Check sheet for the modelled part. Datum: model origin and axes. Units: mm. A direction names the side the tool comes from. Give positions to 0.01 mm unless a question says otherwise; leave off trailing zeros. Write each loop counter-clockwise with the first axis right and the second up, starting at its lowest first coordinate (ties: lowest second). Pieces come first, ordered by that corner, then holes. Notation, with made-up numbers: (-37, -1) -> (-32, -1) arc R10 cw to (-32, 12) -> close; hole circle Ø6 at (65.5, -24). An arc over 180 degrees is marked (long way). Answer as a JSON object with one key per item and string values.
Autodesk Inventor part; units mm, degrees
ref_plane "hhpsjc_r_XY" through (0, 0, 0) normal (0, 1, 0) x (1, 0, 0)
ref_plane "hhpsjc_r_YZ" through (0, 0, 0) normal (1, 0, 0) x (0, 0, -1)
ref_plane "hhpsjc_r_ZX" through (0, 0, 0) normal (0, 0, -1) x (0, 1, 0)
sketch "Sketch_1" plane through (0, 0, 0) normal (0, 0, 1) x (1, 0, 0)
  line L0 (0, -16) -> (0, 16)
  line L1 (0, 16) -> (5, 16)
  line L2 (5, 16) -> (5, -16)
  line L3 (5, -16) -> (0, -16)
  line L4 (0, -16) -> (0, 16)
revolve "Revolution1" add sketch "Sketch_1" angle 360 about axis through (0, -16, 0) along (0, -1, 0)
sketch "Sketch_2" plane through (0, 0, 0) normal (0, 1, 0) x (-1, 0, 0)
  line L0 (0, 1) -> (-16, 1)
  arc A0 (-16, 1) -> (-18, -5) centre (-8, -5) ccw
  line L1 (-18, -5) -> (0, -5)
  line L2 (0, -5) -> (0, 1)
extrude "Extrusion1" add sketch "Sketch_2" along normal mid plane 32
sketch "Sketch_4" plane through (18, 0, 0) normal (1, 0, 0) x (0, 0, -1)
  line L0 (-5, -32) -> (10, -32)
  line L1 (10, -32) -> (10, 32)
  line L2 (10, 32) -> (-5, 32)
  line L3 (-5, 32) -> (-5, -32)
  line L4 (-1, 14) -> (-1, -14)
  arc A0 (-1, -14) -> (5, -16) centre (5, -6) ccw
  line L5 (5, -16) -> (5, 16)
  arc A1 (5, 16) -> (-1, 14) centre (5, 6) ccw
extrude "Extrusion2" cut sketch "Sketch_4" against normal blind 13
sketch "Sketch_6" plane through (0, 0, -5) normal (0, 0, 1) x (1, 0, 0)
  circle A0 centre (10.5, 12) radius 2.75
extrude "Extrusion3" add sketch "Sketch_6" against normal blind 4
sketch "Sketch_5" plane through (0, 0, -5) normal (0, 0, 1) x (1, 0, 0)
  circle A0 centre (10.5, -12) radius 2.75
extrude "Extrusion4" add sketch "Sketch_5" against normal blind 4
sketch "Sketch_7" plane through (10.5, 0, 0) normal (1, 0, 0) x (0, 0, -1)
  line L0 (5, 0) -> (-1, 0)
  line L1 (-1, 0) -> (-1, 5.5)
  line L2 (-1, 5.5) -> (1.75, 2.75)
  line L3 (1.75, 2.75) -> (5, 2.75)
  line L4 (5, 2.75) -> (5, 0)
  line L5 (5, 0) -> (-1, 0)
revolve "Revolution2" cut sketch "Sketch_7" angle 360 about axis through (10.5, 0, -5) along (0, 0, -1)
sketch "Sketch_8" plane through (0, 0, 0) normal (0, 0, 1) x (1, 0, 0)
  line L0 (0, -16) -> (0, 16)
  line L1 (0, 16) -> (2.5, 16)
  line L2 (2.5, 16) -> (2.5, -16)
  line L3 (2.5, -16) -> (0, -16)
  line L4 (0, -16) -> (0, 16)
revolve "Revolution3" cut sketch "Sketch_8" angle 360 about axis through (0, -16, 0) along (0, -1, 0)
sketch "Sketch_3" plane through (0, 0, 0) normal (0, 0, 1) x (1, 0, 0)
  line L0 (-36, -36) -> (36, -36)
  line L1 (36, -36) -> (36, 36)
  line L2 (36, 36) -> (-36, 36)
  line L3 (-36, 36) -> (-36, -36)
  line L4 (-5, -16) -> (14, -16)
  arc A0 (14, -16) -> (18, -12) centre (14, -12) ccw
  line L5 (18, -12) -> (18, 12)
  arc A1 (18, 12) -> (14, 16) centre (14, 12) ccw
  line L6 (14, 16) -> (-5, 16)
  line L7 (-5, 16) -> (-5, 5.5333)
  line L8 (-5, 5.5333) -> (5, 5.5333)
  line L9 (5, 5.5333) -> (5, -5.5333)
  line L10 (5, -5.5333) -> (-5, -5.5333)
  line L11 (-5, -5.5333) -> (-5, -16)
extrude "Extrusion5" cut sketch "Sketch_3" along normal mid plane 10
ref_plane "hhpsjc_r_XY" through (0, 0, 0) normal (0, 1, 0) x (1, 0, 0)
ref_plane "hhpsjc_r_YZ" through (0, 0, 0) normal (1, 0, 0) x (0, 0, -1)
ref_plane "hhpsjc_r_ZX" through (0, 0, 0) normal (0, 0, -1) x (0, 1, 0)
ref_plane "hole2_to_bolt_XY" through (10.5, 0, 1) normal (0, 0, 1) x (1, 0, 0)
ref_plane "hole2_to_bolt_YZ" through (10.5, 0, 1) normal (1, 0, 0) x (0, 1, 0)
ref_plane "hole2_to_bolt_ZX" through (10.5, 0, 1) normal (0, 1, 0) x (0, 0, 1)
ref_plane "nut2_to_bolt_XY" through (10.5, 0, -7) normal (0, 0, 1) x (1, 0, 0)
ref_plane "nut2_to_bolt_YZ" through (10.5, 0, -7) normal (1, 0, 0) x (0, 1, 0)
ref_plane "nut2_to_bolt_ZX" through (10.5, 0, -7) normal (0, 1, 0) x (0, 0, 1)
properties part number "HHPSJC5-r"
1. Mould release check, pull along Y, two halves, no side actions. Record for faces 6 (the face through (2, 16, -2)), 7 (the face through (2, -16, -2)), 8 (the face through (-0.54, -10.84, -2.44)), 9 (the face through (13.35, -0.63, -1.58)): released by +Y, released by -Y, zero draft, split by the parting line, or undercut.
Determined:
{"face 6": "released by +Y", "face 7": "released by -Y", "face 8": "zero draft", "face 9": "undercut"}
2. Sectioned sample at B-B, the plane z = -1. Enter the section's corners in (x, y).
Determined:
{"outline": "(-4.9, -16) -> (-2.29, -16) -> (-2.29, -5.53) -> (-4.9, -5.53) -> close; (-4.9, 5.53) -> (-2.29, 5.53) -> (-2.29, 16) -> (-4.9, 16) -> close; (2.29, -16) -> (5, -16) -> (5, -15.17) -> (16.45, -15.17) arc R4 ccw to (17.17, -14.45) -> (17.17, 14.45) arc R4 ccw to (16.45, 15.17) -> (5, 15.17) -> (5, 16) -> (2.29, 16) -> (2.29, 5.53) -> (5, 5.53) -> (5, -5.53) -> (2.29, -5.53) -> close; hole circle Ø7 at (10.5, 0)"}
3. Sectioned sample at A-A, the plane x = 4. Enter the section's corners in (y, z), plus the area to 3 significant figures.
Determined:
{"outline": "(-16, -5) -> (-5.53, -5) -> (-5.53, 3) -> (-16, 3) -> close; (5.53, -5) -> (16, -5) -> (16, 3) -> (5.53, 3) -> close", "area": "167 mm^2"}
4. Sectioned sample at D-D, the plane x = -1.75. Enter the section's corners in (y, z).
Determined:
{"outline": "(-16, -4.68) -> (-5.53, -4.68) -> (-5.53, -1.79) -> (-16, -1.79) -> close; (-16, 1.79) -> (-5.53, 1.79) -> (-5.53, 4.68) -> (-16, 4.68) -> close; (5.53, -4.68) -> (16, -4.68) -> (16, -1.79) -> (5.53, -1.79) -> close; (5.53, 1.79) -> (16, 1.79) -> (16, 4.68) -> (5.53, 4.68) -> close"}
5. Scan lines: L1, parallel to Z at x = 0, y = 8; L2, parallel to Y at x = -2.5, z = -2.5; L3, parallel to X at y = 0, z = -3.05. Record each from-to range of solid material in increasing order. Write a range as [from, to].
Determined:
{"L1": "[-5, -2.5], [2.5, 5]", "L2": "[-16, -5.53], [5.53, 16]", "L3": "[5, 7.75], [13.25, 17.81]"}
6. Go/stop test with flat-tipped pins: P1, Ø2, axis at x = 7, z = -2, coming from the -Y side; P2, Ø8, axis at x = 0.5, z = 0, coming from the +Y side; P3, Ø3, axis at y = 0, z = -3, coming from the -X side; P4, Ø5.5, axis at x = 9, y = 5.5, coming from the +Z side. Record where each tip stops, or that it passes through.
Determined:
{"P1": "y = -15.8", "P2": "y = 16", "P3": "x = 5", "P4": "z = 1"}
7. Access from +Z, -Z, +X, -X, +Y, -Y to the whole of each face (thin tool, end or side, straight path). Record for faces 1 (the face through (2, -5.533, -2)), 2 (the face through (5, -15, 0)), 3 (the face through (7, 0, -5)), 4 (the face through (10, -10, 1)), 5 (the face through (11, 15.5, -1.88)).
Determined:
{"face 1": "+Z, -Z, -X", "face 2": "+Z, +X, -Y", "face 3": "-Z", "face 4": "+Z, +X, +Y, -Y", "face 5": "+Z, +X, +Y"}
8. Sectioned sample at C-C, the plane z = 3.75. Enter the section's corners in (x, y).
Determined:
{"outline": "(-3.31, -16) -> (3.31, -16) -> (3.31, -5.53) -> (-3.31, -5.53) -> close; (-3.31, 5.53) -> (3.31, 5.53) -> (3.31, 16) -> (-3.31, 16) -> close"}
